Autodesk Inventor part; units mm, degrees
ref_plane "YZ Plane" through (0, 0, 0) normal (1, 0, 0) x (0, 1, 0)
ref_plane "XZ Plane" through (0, 0, 0) normal (0, 1, 0) x (-1, 0, 0)
ref_plane "XY Plane" through (0, 0, 0) normal (0, 0, 1) x (1, 0, 0)
sketch "Sketch1" plane through (0, 0, 0) normal (0, 0, 1) x (1, 0, 0)
  line L0 (-36.9381, 4.4529) -> (64.6619, 4.4529)
  line L1 (64.6619, 4.4529) -> (64.6619, -14.5971)
  line L2 (64.6619, -14.5971) -> (-36.9381, -14.5971)
  line L3 (-36.9381, -14.5971) -> (-36.9381, 4.4529)
  point P0 (0, 0)
  dimension "d0" = 101.6
  dimension "d1" = 19.05
extrude "Extrusion1" add sketch "Sketch1" along normal blind 7.9375
sketch "Sketch2" plane through (0, 0, 7.9375) normal (0, 0, 1) x (1, 0, 0)
  line L0 (-36.9381, -14.5971) -> (-36.9381, 4.4529)
  line L1 (64.6619, -14.5971) -> (-36.9381, -14.5971)
  line L2 (-36.9381, -5.0721) -> (13.8619, -5.0721)
  line L3 (13.8619, -5.0721) -> (58.6929, -5.0721)
  line L4 (58.6929, -5.0721) -> (-30.9691, -5.0721)
  circle A0 centre (-30.9691, -5.0721) radius 1.9812
  circle A1 centre (58.6929, -5.0721) radius 1.9812
  point P0 (0, 0)
  dimension "d4" = 44.831
  dimension "d5" = 89.662
  dimension "d6" = 3.9624
extrude "Extrusion2" cut sketch "Sketch2" against normal blind 7.9375
properties part number "spacers"
The listing builds one solid part. Answer for the finished solid, in the listing's coordinates (mm). Round coordinates to 2 decimals unless told otherwise and drop trailing zeros. Use one line per item in the form item = value. Start each with the question number.
1. Given pin 1 Ø3 at (x, y) = (58.69, -5.07) entering from +Z, flat-ended and moving along its own axis, determine where the tip first touches the part or whether it passes through.
2. For a pull along Y with two mould halves and no side action, classify faces 1 (the face through (64.662, -5, 4)), 2 (the face through (15, -14.597, 4)), 3 (the face through (-32.95, -4.98, 4.02)) as pulls with the +Y half, pulls with the -Y half, needs draft (parallel to the pull), parting line crosses it, or undercut.
3. Consider line 1 (X direction, y = -4.5, z = 2); line 2 (X direction, y = -3.75, z = 3.5); line 3 (Y direction, x = -30.5, z = 5.75). Determine where each line is inside the solid, lowest interval first. Write a range as [from, to].
Geometry check:
q1.pin_1 = through
q2.face_1 = needs draft
q2.face_2 = pulls with the -Y half
q2.face_3 = undercut
q3.line_1 = [-36.94, -32.87], [-29.07, 56.8], [60.59, 64.66]
q3.line_2 = [-36.94, -32.44], [-29.49, 57.22], [60.17, 64.66]
q3.line_3 = [-14.6, -7], [-3.15, 4.45]
